Geometry check sheet. Reference: the model listing, model coordinates, mm. Face numbers are marked on the shaded views. A direction names the side the tool comes from. Coordinates: 2 decimals unless noted, no trailing zeros. Write each loop counter-clockwise with the first axis right and the second up, starting at its lowest first coordinate (ties: lowest second). Pieces come first, ordered by that corner, then holes. Notation, with made-up numbers: (27, -13) -> (60, -13) arc R25 cw to (60, 20) -> close; hole circle Ø10 at (87, 9.25). An arc over 180 degrees is marked (long way). Use a Markdown table: item, result.
```python
from build123d import *

# Parameters (mm, degrees)
BOSS_EXTRUDE1_DEPTH = 8
CUT_EXTRUDE1_REACH  = 32.136
SKETCH2_R           = 1.5
CUT_EXTRUDE2_REACH  = 31.156
SKETCH3_R           = 1.5
CUT_EXTRUDE3_REACH  = 28.908
SKETCH4_R           = 1.5
SKETCH5_R           = 4.5
CUT_EXTRUDE4_DEPTH  = 5
SKETCH6_R           = 1.5
CUT_EXTRUDE5_DEPTH  = 26.183317902
FILLET1_R           = 4


with BuildPart() as part:
    # Sketch1 → Boss-Extrude1 (new body)
    with BuildSketch(Plane(origin=(0, 0, 0), x_dir=(1, 0, 0), z_dir=(0, 1, 0))):
        with BuildLine():
            ThreePointArc((-2.946152423, -6.897114317), (-3.95544326, -6.372163574), (-4.873724357, -5.700597415))
            Line((-4.873724357, -5.700597415), (-13.905444566, -10.915063509))
            Line((-13.905444566, -10.915063509), (-12.905444566, -12.647114317))
            Line((-12.905444566, -12.647114317), (-2.946152423, -6.897114317))
        make_face()
        with BuildLine():
            Line((-16.405444566, -6.584936491), (-7.373724357, -1.370470396))
            ThreePointArc((-7.373724357, -1.370470396), (-7.496177162, -0.23943256), (-7.446152423, 0.897114317))
            Line((-7.446152423, 0.897114317), (-17.405444566, -4.852885683))
            Line((-17.405444566, -4.852885683), (-16.405444566, -6.584936491))
        make_face()
        Polygon((-2.5, 1.443375673), (-2.5, 0), (0, 0), (-1.25, 2.165063509), align=None)
        Polygon((1.25, -2.165063509), (0, 0), (-1.25, -2.165063509), (0, -2.886751346), align=None)
        with BuildLine():
            Line((-7.446152423, 0.897114317), (-4.5, 2.598076211))
            Line((-4.5, 2.598076211), (-4.5, 6))
            ThreePointArc((-4.5, 6), (-6.495190528, 3.75), (-7.446152423, 0.897114317))
        make_face()
        with BuildLine():
            Line((0, -5.196152423), (-2.946152423, -6.897114317))
            ThreePointArc((-2.946152423, -6.897114317), (0, -7.5), (2.946152423, -6.897114317))
            Line((2.946152423, -6.897114317), (0, -5.196152423))
        make_face()
        Polygon((1.25, 2.165063509), (0, 0), (2.5, 0), (2.5, 1.443375673), align=None)
        with BuildLine():
            ThreePointArc((7.446152423, 0.897114317), (6.495190528, 3.75), (4.5, 6))
            Line((4.5, 6), (4.5, 2.598076211))
            Line((4.5, 2.598076211), (7.446152423, 0.897114317))
        make_face()
        with BuildLine():
            ThreePointArc((7.5, 0), (7.468364368, -0.688137822), (7.373724357, -1.370470396))
            Line((7.373724357, -1.370470396), (16.405444566, -6.584936491))
            Line((16.405444566, -6.584936491), (17.405444566, -4.852885683))
            Line((17.405444566, -4.852885683), (7.446152423, 0.897114317))
            ThreePointArc((7.446152423, 0.897114317), (7.486526002, 0.449364457), (7.5, 0))
        make_face()
        with BuildLine():
            ThreePointArc((4.873724357, -5.700597415), (3.95544326, -6.372163574), (2.946152423, -6.897114317))
            Line((2.946152423, -6.897114317), (12.905444566, -12.647114317))
            Line((12.905444566, -12.647114317), (13.905444566, -10.915063509))
            Line((13.905444566, -10.915063509), (4.873724357, -5.700597415))
        make_face()
        with BuildLine():
            Line((2.5, 17.5), (2.5, 7.071067812))
            ThreePointArc((2.5, 7.071067812), (3.540733902, 6.611596134), (4.5, 6))
            Line((4.5, 6), (4.5, 17.5))
            Line((4.5, 17.5), (2.5, 17.5))
        make_face()
        with BuildLine():
            Line((-4.5, 17.5), (-4.5, 6))
            ThreePointArc((-4.5, 6), (-3.540733902, 6.611596134), (-2.5, 7.071067812))
            Line((-2.5, 7.071067812), (-2.5, 17.5))
            Line((-2.5, 17.5), (-4.5, 17.5))
        make_face()
        with BuildLine():
            Line((-2.5, 0), (-4.5, 0))
            Line((-4.5, 0), (-4.5, 0.288675135))
            Line((-4.5, 0.288675135), (-7.373724357, -1.370470396))
            ThreePointArc((-7.373724357, -1.370470396), (-6.495190528, -3.75), (-4.873724357, -5.700597415))
            Line((-4.873724357, -5.700597415), (-2, -4.041451884))
            Line((-2, -4.041451884), (-2.25, -3.897114317))
            Line((-2.25, -3.897114317), (-1.25, -2.165063509))
            Line((-1.25, -2.165063509), (0, 0))
            Line((0, 0), (-2.5, 0))
        make_face()
        Polygon((-4.5, 0.288675135), (-4.5, 0), (-2.5, 0), (-2.5, 1.443375673), align=None)
        with BuildLine():
            Line((-7.373724357, -1.370470396), (-4.5, 0.288675135))
            Line((-4.5, 0.288675135), (-4.5, 2.598076211))
            Line((-4.5, 2.598076211), (-7.446152423, 0.897114317))
            ThreePointArc((-7.446152423, 0.897114317), (-7.496177162, -0.23943256), (-7.373724357, -1.370470396))
        make_face()
        Polygon((-4.5, 2.598076211), (-4.5, 0.288675135), (-2.5, 1.443375673), (-2.5, 3.75277675), align=None)
        with BuildLine():
            Line((-4.5, 6), (-4.5, 2.598076211))
            Line((-4.5, 2.598076211), (-2.5, 3.75277675))
            Line((-2.5, 3.75277675), (-2.5, 7.071067812))
            ThreePointArc((-2.5, 7.071067812), (-3.540733902, 6.611596134), (-4.5, 6))
        make_face()
        Polygon((-2.5, 3.75277675), (-2.5, 1.443375673), (-1.25, 2.165063509), (-2.25, 3.897114317), align=None)
        with BuildLine():
            Line((2.5, 0), (0, 0))
            Line((0, 0), (1.25, -2.165063509))
            Line((1.25, -2.165063509), (2.25, -3.897114317))
            Line((2.25, -3.897114317), (2, -4.041451884))
            Line((2, -4.041451884), (4.873724357, -5.700597415))
            ThreePointArc((4.873724357, -5.700597415), (6.495190528, -3.75), (7.373724357, -1.370470396))
            Line((7.373724357, -1.370470396), (4.5, 0.288675135))
            Line((4.5, 0.288675135), (4.5, 0))
            Line((4.5, 0), (2.5, 0))
        make_face()
        with BuildLine():
            Line((-1.25, 2.165063509), (0, 0))
            Line((0, 0), (1.25, 2.165063509))
            Line((1.25, 2.165063509), (2.25, 3.897114317))
            Line((2.25, 3.897114317), (2.5, 3.75277675))
            Line((2.5, 3.75277675), (2.5, 7.071067812))
            ThreePointArc((2.5, 7.071067812), (0, 7.5), (-2.5, 7.071067812))
            Line((-2.5, 7.071067812), (-2.5, 3.75277675))
            Line((-2.5, 3.75277675), (-2.25, 3.897114317))
            Line((-2.25, 3.897114317), (-1.25, 2.165063509))
        make_face()
        with BuildLine():
            Line((-2, -4.041451884), (-4.873724357, -5.700597415))
            ThreePointArc((-4.873724357, -5.700597415), (-3.95544326, -6.372163574), (-2.946152423, -6.897114317))
            Line((-2.946152423, -6.897114317), (0, -5.196152423))
            Line((0, -5.196152423), (-2, -4.041451884))
        make_face()
        Polygon((2.5, 1.443375673), (2.5, 0), (4.5, 0), (4.5, 0.288675135), align=None)
        Polygon((2.25, -3.897114317), (1.25, -2.165063509), (0, -2.886751346), (2, -4.041451884), align=None)
        Polygon((2.25, 3.897114317), (1.25, 2.165063509), (2.5, 1.443375673), (2.5, 3.75277675), align=None)
        Polygon((0, -2.886751346), (-1.25, -2.165063509), (-2.25, -3.897114317), (-2, -4.041451884), align=None)
        Polygon((0, -2.886751346), (-2, -4.041451884), (0, -5.196152423), (2, -4.041451884), align=None)
        Polygon((2.5, 3.75277675), (2.5, 1.443375673), (4.5, 0.288675135), (4.5, 2.598076211), align=None)
        with BuildLine():
            ThreePointArc((4.5, 6), (3.540733902, 6.611596134), (2.5, 7.071067812))
            Line((2.5, 7.071067812), (2.5, 3.75277675))
            Line((2.5, 3.75277675), (4.5, 2.598076211))
            Line((4.5, 2.598076211), (4.5, 6))
        make_face()
        with BuildLine():
            Line((2, -4.041451884), (0, -5.196152423))
            Line((0, -5.196152423), (2.946152423, -6.897114317))
            ThreePointArc((2.946152423, -6.897114317), (3.95544326, -6.372163574), (4.873724357, -5.700597415))
            Line((4.873724357, -5.700597415), (2, -4.041451884))
        make_face()
        with BuildLine():
            Line((4.5, 2.598076211), (4.5, 0.288675135))
            Line((4.5, 0.288675135), (7.373724357, -1.370470396))
            ThreePointArc((7.373724357, -1.370470396), (7.468364368, -0.688137822), (7.5, 0))
            ThreePointArc((7.5, 0), (7.486526002, 0.449364457), (7.446152423, 0.897114317))
            Line((7.446152423, 0.897114317), (4.5, 2.598076211))
        make_face()
    extrude(amount=BOSS_EXTRUDE1_DEPTH)

    # Cut-Extrude1: up to this face of the body (flat: up to its plane)
    cut_extrude1_end = Plane(part.part.faces().sort_by_distance((-12.425798494, 4, 1.977885683))[0])
    # Sketch2 → Cut-Extrude1 (cut, up to the picked face)
    with BuildSketch(Plane(origin=(2.25, 0, 3.897114317), x_dir=(0.8660254037844364, 0, -0.5000000000000039), z_dir=(0.5000000000000039, 0, 0.8660254037844364)), mode=Mode.PRIVATE) as cut_extrude1_sk1:
        with Locations((-13, 4)):
            Circle(SKETCH2_R)
    cut_extrude1_tool1 = split(extrude(cut_extrude1_sk1.sketch, amount=-CUT_EXTRUDE1_REACH, mode=Mode.PRIVATE), bisect_by=cut_extrude1_end, keep=Keep.BOTH, mode=Mode.PRIVATE)
    add(cut_extrude1_tool1.solids().sort_by(Axis((-9.00833, 4, 10.397114), (-0.5000000000000039, 0, -0.8660254037844364)))[0], mode=Mode.SUBTRACT)

    # Cut-Extrude2: up to this face of the body (flat: up to its plane)
    cut_extrude2_end = Plane(part.part.faces().sort_by_distance((4.5, 4, -11.75))[0])
    # Sketch3 → Cut-Extrude2 (cut, up to the picked face)
    with BuildSketch(Plane.ZY.offset(4.5), mode=Mode.PRIVATE) as cut_extrude2_sk1:
        with Locations((-13, 4)):
            Circle(SKETCH3_R)
    cut_extrude2_tool1 = split(extrude(cut_extrude2_sk1.sketch, amount=-CUT_EXTRUDE2_REACH, mode=Mode.PRIVATE), bisect_by=cut_extrude2_end, keep=Keep.BOTH, mode=Mode.PRIVATE)
    add(cut_extrude2_tool1.solids().sort_by(Axis((-4.5, 4, -13), (1, 0, 0)))[0], mode=Mode.SUBTRACT)

    # Cut-Extrude3: up to this face of the body (flat: up to its plane)
    cut_extrude3_end = Plane(part.part.faces().sort_by_distance((7.925798494, 4, 9.772114317))[0])
    # Sketch4 → Cut-Extrude3 (cut, up to the picked face)
    with BuildSketch(Plane(origin=(2.25, 0, -3.897114317), x_dir=(-0.8660254037844363, 0, -0.5000000000000042), z_dir=(0.5000000000000041, 0, -0.8660254037844362)), mode=Mode.PRIVATE) as cut_extrude3_sk1:
        with Locations((-13, 4)):
            Circle(SKETCH4_R)
    cut_extrude3_tool1 = split(extrude(cut_extrude3_sk1.sketch, amount=-CUT_EXTRUDE3_REACH, mode=Mode.PRIVATE), bisect_by=cut_extrude3_end, keep=Keep.BOTH, mode=Mode.PRIVATE)
    add(cut_extrude3_tool1.solids().sort_by(Axis((13.50833, 4, 2.602886), (-0.5000000000000041, 0, 0.8660254037844362)))[0], mode=Mode.SUBTRACT)

    # Sketch5 → Cut-Extrude4 (cut)
    with BuildSketch(Plane.XZ):
        with Locations(Location((0, 0, 0), (0, 0, 270))):
            Circle(SKETCH5_R)
    extrude(amount=-CUT_EXTRUDE4_DEPTH, mode=Mode.SUBTRACT)

    # Sketch6 → Cut-Extrude5 (cut, through all)
    with BuildSketch(Plane.XZ.offset(-5)):
        with Locations(Location((0, 0, 0), (0, 0, 270))):
            Circle(SKETCH6_R)
    extrude(amount=-CUT_EXTRUDE5_DEPTH, mode=Mode.SUBTRACT)

    # Fillet1
    fillet1_edges = [part.edges().sort_by_distance(p)[0] for p in [
        (-13.405444566, 0, 11.781088913),
        (-13.405444566, 8, 11.781088913),
        (-16.905444566, 0, 5.718911087),
        (-16.905444566, 8, 5.718911087),
        (-3.5, 0, -17.5),
        (-3.5, 8, -17.5),
        (3.5, 0, -17.5),
        (3.5, 8, -17.5),
        (13.405444566, 0, 11.781088913),
        (13.405444566, 8, 11.781088913),
        (16.905444566, 0, 5.718911087),
        (16.905444566, 8, 5.718911087),
    ]]
    fillet(fillet1_edges, radius=FILLET1_R - 0.0001)  # a hair under: the kernel refuses the full size


solid = part.part
```
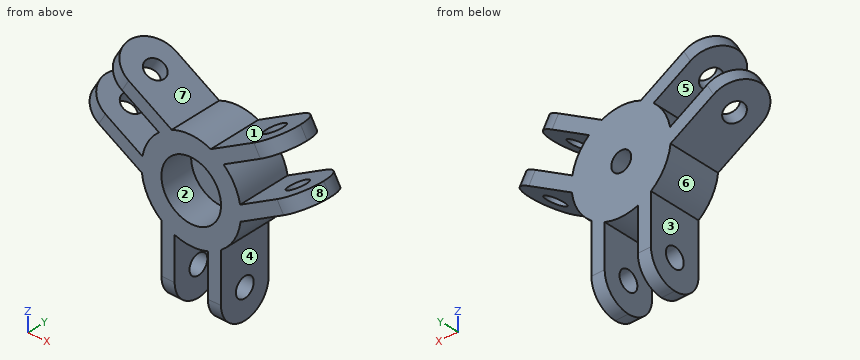
Item 1: Depth check by flat-ended pin: P1, Ø1, axis at x = 8, y = 6.5, coming from the -Z side; P2, Ø1, axis at y = 1.5, z = 9.5, coming from the -X side; P3, Ø3, axis at x = 12, y = 3.5, coming from the -Z side. Enter the tip coordinate at first touch or a pass-through.
Answer block:
| item | result |
|---|---|
| P1 | stops at z = -0.87 |
| P2 | stops at x = -12.32 |
| P3 | stops at z = 0.87 |
Item 2: Thickness scan on L1, parallel to X at y = 6, z = -11; L2, parallel to X at y = 2.2, z = 0; L3, parallel to Y at x = -3, z = -13. Record the ranges inside material, lowest first. Write a range as [from, to].
Answer block:
| item | result |
|---|---|
| L1 | x = [-4.5, -2.5], [2.5, 4.5] |
| L2 | x = [-9, -4.5], [4.5, 9] |
| L3 | y = [0, 2.5], [5.5, 8] |
Item 3: Section check B-B on z = 0. Record the boundary of the cut face in (x, y), then the cut area to 3 significant figures.
Answer block:
| item | result |
|---|---|
| outline | (-9, 0) -> (-4.5, 0) -> (-4.5, 5) -> (-1.5, 5) -> (-1.5, 8) -> (-9, 8) -> close; (1.5, 5) -> (4.5, 5) -> (4.5, 0) -> (9, 0) -> (9, 8) -> (1.5, 8) -> close |
| area | 90.0 mm^2 |
Item 4: Mould release check, pull along X, two halves, no side actions. Record for the marked faces 6, 7 and 8: +X half, -X half, draft (parallel to the pull), parting line (faces both ways), or undercut.
Answer block:
| item | result |
|---|---|
| face 6 | -X half |
| face 7 | undercut |
| face 8 | +X half |
Item 5: Section check C-C on z = -13. Record the boundary of the cut face in (x, y), then the cut area to 3 significant figures.
Answer block:
| item | result |
|---|---|
| outline | (-4.5, 0) -> (-2.5, 0) -> (-2.5, 2.5) -> (-4.5, 2.5) -> close; (-4.5, 5.5) -> (-2.5, 5.5) -> (-2.5, 8) -> (-4.5, 8) -> close; (2.5, 0) -> (4.5, 0) -> (4.5, 2.5) -> (2.5, 2.5) -> close; (2.5, 5.5) -> (4.5, 5.5) -> (4.5, 8) -> (2.5, 8) -> close |
| area | 20.0 mm^2 |
Item 6: Tool access check on the marked faces 1, 2, 3, 4 and 5. Record the directions out of +Z, -Z, +X, -X, +Y, -Y that give a thin tool (end or side, any length) a straight path to the whole face; none if there is none.
Answer block:
| item | result |
|---|---|
| face 1 | +Z, +Y, -Y |
| face 2 | -Y |
| face 3 | -Z, -X, +Y, -Y |
| face 4 | -Z, +X, +Y, -Y |
| face 5 | +Y, -Y |
Item 7: Section check D-D on y = 7.5. Record the boundary of the cut face in (x, z), then the cut area to 3 significant figures.
Answer block:
| item | result |
|---|---|
| outline | (-15.62, 3.82) -> (-7.45, -0.9) arc R7.5 ccw to (-4.5, -6) -> (-4.5, -15.44) -> (-2.5, -15.44) -> (-2.5, -7.07) arc R7.5 ccw to (2.5, -7.07) -> (2.5, -15.44) -> (4.5, -15.44) -> (4.5, -6) arc R7.5 ccw to (7.45, -0.9) -> (15.62, 3.82) -> (14.62, 5.55) -> (7.37, 1.37) arc R7.5 ccw to (4.87, 5.7) -> (12.12, 9.88) -> (11.12, 11.62) -> (2.95, 6.9) arc R7.5 ccw to (-2.95, 6.9) -> (-11.12, 11.62) -> (-12.12, 9.88) -> (-4.87, 5.7) arc R7.5 ccw to (-7.37, 1.37) -> (-14.62, 5.55) -> close; hole circle Ø3 at (0, 0) |
| area | 276 mm^2 |
Item 8: Section check A-A on x = 0. Record the boundary of the cut face in (y, z), then the cut area to 3 significant figures.
Answer block:
| item | result |
|---|---|
| outline | (0, -7.5) -> (8, -7.5) -> (8, -1.5) -> (5, -1.5) -> (5, -4.5) -> (0, -4.5) -> close; (0, 4.5) -> (5, 4.5) -> (5, 1.5) -> (8, 1.5) -> (8, 7.5) -> (0, 7.5) -> close |
| area | 66.0 mm^2 |
